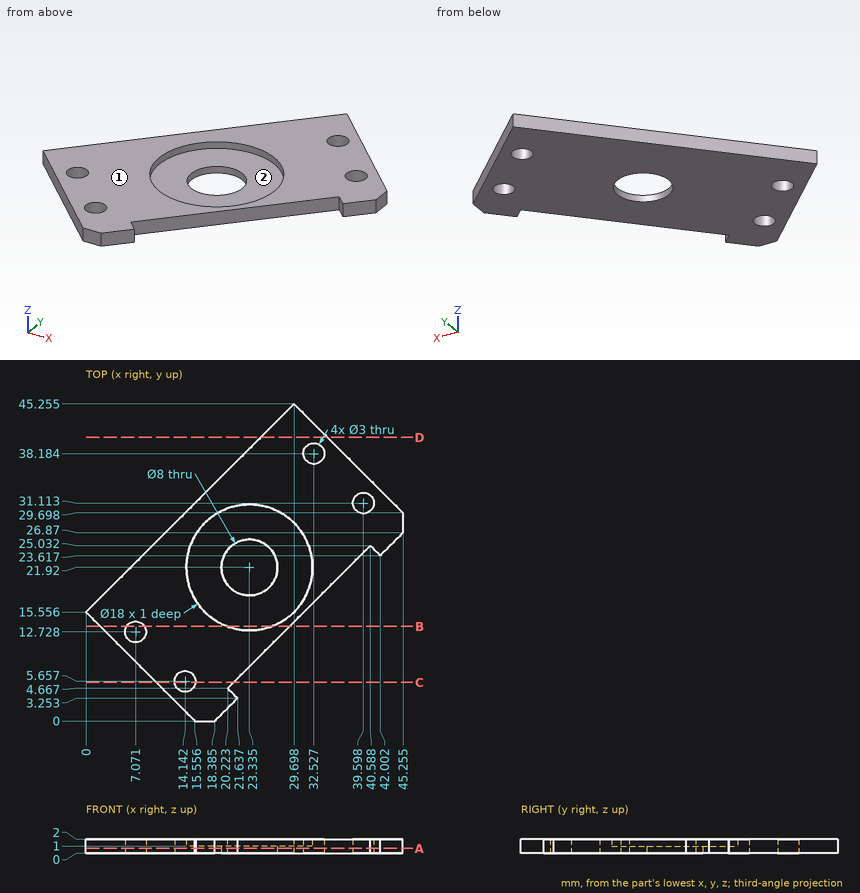
The drawing under review shows one solid part. Ordinate dimensions are in mm from its lowest x, y, z. A direction names the side the tool comes from. Round coordinates to 2 decimals unless told otherwise and drop trailing zeros. Write each loop counter-clockwise with the first axis right and the second up, starting at its lowest first coordinate (ties: lowest second). Pieces come first, ordered by that corner, then holes. Notation, with made-up numbers: (1.5, 76) -> (51.5, 76) arc R17 cw to (51.5, 97) -> close; hole circle Ø3 at (10.25, 30). An arc over 180 degrees is marked (long way). One line per question, with ' | ' between items.
(1) Take a section at D-D, the plane y = 40.5. State the section outline as (x, z) points.
Result sheet:
outline: (24.94, 0) -> (34.45, 0) -> (34.45, 2) -> (24.94, 2) -> close
(2) Insertion check: P1, Ø11, axis at x = 23.33, y = 21.92, coming from the +Z side. The pin has a flat end and moves straight along its axis. Give the tip position at first contact, or say it passes through.
Result sheet:
P1: z = 1
(3) Take a section at C-C, the plane y = 5.5. State the section outline as (x, z) points.
Result sheet:
outline: (10.06, 0) -> (12.65, 0) -> (12.65, 2) -> (10.06, 2) -> close; (15.63, 0) -> (21.06, 0) -> (21.06, 2) -> (15.63, 2) -> close
(4) Wall thickness on line 1 (X direction, y = 24, z = 1.65) (1 decimal); line 2 (Y direction, x = 24, z = 1.3) (1 decimal); line 3 (X direction, y = 39, z = 1.8) (1 decimal): over which ranges is each line inside the solid? List them lowest first. Write a range as [from, to].
Result sheet:
line 1: [8.4, 14.6], [32.1, 39.6], [41.6, 42.4] | line 2: [8.4, 12.9], [30.9, 39.6] | line 3: [23.4, 31.3], [33.8, 36]
(5) Take a section at B-B, the plane y = 13.5. State the section outline as (x, z) points (1 decimal).
Result sheet:
outline: (2.1, 0) -> (5.8, 0) -> (5.8, 2) -> (2.1, 2) -> close; (8.4, 0) -> (29.1, 0) -> (29.1, 2) -> (26.5, 2) -> (26.5, 1) -> (20.2, 1) -> (20.2, 2) -> (8.4, 2) -> close
(6) Machinability: for the marked faces 1 and 2, which of the approach directions +Z, -Z, +X, -X, +Y, -Y give a long, thin tool a straight path to every point of the face, cutting with its end or side? Answer none if there is none.
Result sheet:
face 1: +Z, +X, -X, +Y, -Y | face 2: +Z
(7) Take a section at A-A, the plane z = 0.65. State the section outline as (x, y) points (1 decimal).
Result sheet:
outline: (0, 15.6) -> (15.6, 0) -> (18.4, 0) -> (21.6, 3.3) -> (20.2, 4.7) -> (40.6, 25) -> (42, 23.6) -> (45.3, 26.9) -> (45.3, 29.7) -> (29.7, 45.3) -> close; hole circle Ø3 at (7.1, 12.7); hole circle Ø3 at (14.1, 5.7); hole circle Ø8 at (23.3, 21.9); hole circle Ø3 at (32.5, 38.2); hole circle Ø3 at (39.6, 31.1)
